Verification items for the finished model (mm, model axes). A direction names the side the tool comes from. Coordinates: 2 decimals unless noted, no trailing zeros. Write each loop counter-clockwise with the first axis right and the second up, starting at its lowest first coordinate (ties: lowest second). Pieces come first, ordered by that corner, then holes. Notation, with made-up numbers: (-7, 10.25) - (23, 10.25) arc R30 cw to (23, 48.25) - close; hole circle Ø9 at (47, 34). An arc over 180 degrees is marked (long way). Use one line per item in the form item = value. Start each with the question number.
(1) Sectioned sample at D-D (x = 6). Record the cut outline in (y, z).
(2) Mould release check, pull along Y, two halves, no side actions. Record for faces 1 (the flat face through (12.7, 53, 6)), 2 (the flat face through (0, 85.591, 6)), 3 (the cylindrical face through (13.244, -5.491, 6.261)): released by +Y, released by -Y, zero draft, split by the parting line, or undercut.
(3) Sectioned sample at A-A (x = 0). Record the cut outline in (y, z), and give its area (3 significant figures).
(4) Sectioned sample at B-B (z = 1.25). Record the cut outline in (x, y), and give its area (3 significant figures).
(5) Sectioned sample at C-C (y = 62). Record the cut outline in (x, z).
(6) Material ranges on line 1 (Y direction, x = 0, z = 6.25); line 2 (X direction, y = 77, z = 5.75); line 3 (X direction, y = -0.5, z = 8.75), recorded low to high. Write a range as [from, to].
(7) Gauge pin test, flat ends, axial feed: pin 1 Ø6.5 at (y, z) = (43.5, 8.5) entering from -X; pin 2 Ø1.5 at (x, z) = (-11, 1.5) entering from -Y; pin 3 Ø2 at (y, z) = (-1.5, 4) entering from +X. Record the tip position at first contact, or that the pin passes through.
(8) Tool access check on faces 4 (the flat face through (0, 31, 12.7)), 5 (the flat face through (-12.7, 54, 6)). Record the directions out of +Z, -Z, +X, -X, +Y, -Y that give a thin tool (end or side, any length) a straight path to the whole face; none if there is none.
from build123d import *

# Parameters (mm, degrees)
F0_R     = 14.3372968019
F1_DEPTH = 12.7


# Not quite as in the source:
# - a feature names something its author has since deleted; it is built from what else it names


with BuildPart() as f1:
    # F0 (on Top) → F1 (new body)
    with BuildSketch(Plane.XY):
        with BuildLine():
            ThreePointArc((-12.7, 21.9970452561), (0, 25.4), (12.7, 21.9970452561))
            Line((12.7, 21.9970452561), (12.7, 85.5907872319))
            Line((12.7, 85.5907872319), (0, 85.5907872319))
            Line((0, 85.5907872319), (-12.7, 85.5907872319))
            Line((-12.7, 85.5907872319), (-12.7, 21.9970452561))
        make_face()
        with BuildLine():
            ThreePointArc((-12.7, 21.9970452561), (-12.7, -21.9970452561), (25.4, 0))
            ThreePointArc((25.4, 0), (21.9970452561, 12.7), (12.7, 21.9970452561))
            ThreePointArc((12.7, 21.9970452561), (0, 25.4), (-12.7, 21.9970452561))
        make_face()
        Circle(F0_R, mode=Mode.SUBTRACT)
    extrude(amount=F1_DEPTH)


solid = f1.part
Answers below:
q1.outline = (-24.68, 0) - (-13.02, 0) - (-13.02, 12.7) - (-24.68, 12.7) - close; (13.02, 0) - (85.59, 0) - (85.59, 12.7) - (13.02, 12.7) - close
q2.face_1 = zero draft
q2.face_2 = released by +Y
q2.face_3 = undercut
q3.outline = (-25.4, 0) - (-14.34, 0) - (-14.34, 12.7) - (-25.4, 12.7) - close; (14.34, 0) - (85.59, 0) - (85.59, 12.7) - (14.34, 12.7) - close
q3.area = 1,050 mm2
q4.outline = (-12.7, 22) arc R25.4 ccw (long way) to (12.7, 22) - (12.7, 85.59) - (-12.7, 85.59) - close; hole circle Ø28.67 at (0, 0)
q4.area = 2,940 mm2
q5.outline = (-12.7, 0) - (12.7, 0) - (12.7, 12.7) - (-12.7, 12.7) - close
q6.line_1 = [-25.4, -14.34], [14.34, 85.59]
q6.line_2 = [-12.7, 12.7]
q6.line_3 = [-25.4, -14.33], [14.33, 25.4]
q7.pin_1 = -12.7
q7.pin_2 = -23.24
q7.pin_3 = 25.4
q8.face_4 = +Z, +X, -X, +Y, -Y
q8.face_5 = +Z, -Z, -X, +Y
